Check sheet for the modelled part. Datum: model origin and axes. Units: mm. A direction names the side the tool comes from. Give positions to 0.01 mm unless a question says otherwise; leave off trailing zeros. Write each loop counter-clockwise with the first axis right and the second up, starting at its lowest first coordinate (ties: lowest second). Pieces come first, ordered by that corner, then holes. Notation, with made-up numbers: (30.5, 75.5) -> (42.5, 75.5) arc R21 ccw to (42.5, 88.5) -> close; hole circle Ø4 at (21, 84.25). An arc over 180 degrees is marked (long way). Use a Markdown table: item, result. Add a question column.
1. Cross-section at A-A (x = 15.24). Enter the section's corners in (y, z) (1 decimal).
2. Release check for a two-part mould opening along Y. For faces 1 (the flat face through (15, -3, -0.159)), 2 (the cylindrical face through (0.267, 4.845, 1.526)), 3 (the flat face through (-10.16, 0, 0)) record: released by +Y, released by -Y, zero draft, split by the parting line, or undercut.
3. Scan lines: probe 1 along X at (y, z) = (0, 3.95); probe 2 along X at (y, z) = (-1.9, 0); probe 3 along Z at (x, y) = (17.5, 2.25). Record each from-to range of solid material in increasing order. Write a range as [from, to].
4. Gauge pin test, flat ends, axial feed: P1, Ø4, axis at x = 16.5, y = -3.5, coming from the +Z side; P2, Ø0.6, axis at x = -16.5, y = 0.5, coming from the -Z side; P3, Ø2, axis at x = 10.5, y = -2.5, coming from the -Z side. Record the tip position at first contact, or that the pin passes through.
5. Cross-section at C-C (z = 2.5). Enter the section's corners in (x, y).
6. Set-up check for faces 4 (the flat face through (15, 3, 0.159)), 5 (the flat face through (-14.67, 0.01, -0.891)), 6 (the flat face through (19.05, 0, -3)), 7 (the cylindrical face through (15.187, 0.54, -1.493)): record each of +Z, -Z, +X, -X, +Y, -Y from which the full face is reachable in a straight line by a thin tool's end or side.
7. Cross-section at B-B (y = 2.5). Enter the section's corners in (x, z).
8. Cross-section at D-D (x = 3). Enter the section's corners in (y, z), then the cut area to 3 significant figures.
from build123d import *

# Parameters (mm, degrees)
F0_R      = 5.08
F1_DEPTH  = 19.05
F3_D      = 3.175
F3_DEPTH  = 7.62
F3_TIP    = 0.9538662327
F4_W      = 2.1017943509
F4_H      = 1.7811305588
F5_DEPTH  = 8.89
F7_DEPTH  = 7.62
F9_R      = 0.396875
F10_DEPTH = 17.781
F12_R     = 0.396875
F13_DEPTH = 25.4


with BuildPart() as f1:
    # F0 (on Right) → F1 (new body, symmetric)
    with BuildSketch(Plane.YZ):
        Circle(F0_R)
    extrude(amount=F1_DEPTH, both=True)

    # F3
    with Locations(Plane.YZ.offset(19.05)):
        with Locations((0, 0)):
            Hole(F3_D / 2, depth=F3_DEPTH)
            with Locations((0, 0, -(F3_DEPTH + F3_TIP / 2))):  # 118° drill point
                Cone(0, F3_D / 2, F3_TIP, mode=Mode.SUBTRACT)

    # F4 (on face) → F5 (cut)
    with BuildSketch(Plane(origin=(-19.05, 0, 0), x_dir=(0, -1, 0), z_dir=(-1, 0, 0))):
        Rectangle(F4_W, F4_H)
    extrude(amount=-F5_DEPTH, mode=Mode.SUBTRACT)

    # F6 (on face) → F7 (cut)
    with BuildSketch(Plane.YZ.offset(19.05)):
        with BuildLine():
            ThreePointArc((5.08, 0), (5.0793796935, 0.0793846935), (5.0775189254, 0.15875))
            Line((5.0775189254, 0.15875), (1.5795425564, 0.15875))
            ThreePointArc((1.5795425564, 0.15875), (1.5855093911, 0.0794746554), (1.5875, 0))
            ThreePointArc((1.5875, 0), (1.5855093911, -0.0794746554), (1.5795425564, -0.15875))
            Line((1.5795425564, -0.15875), (5.0775189254, -0.15875))
            ThreePointArc((5.0775189254, -0.15875), (5.0793796935, -0.0793846935), (5.08, 0))
        make_face()
        with BuildLine():
            Line((-1.5795425564, 0.15875), (-5.0775189254, 0.15875))
            ThreePointArc((-5.0775189254, 0.15875), (-5.08, 0), (-5.0775189254, -0.15875))
            Line((-5.0775189254, -0.15875), (-1.5795425564, -0.15875))
            ThreePointArc((-1.5795425564, -0.15875), (-1.5875, 0), (-1.5795425564, 0.15875))
        make_face()
    extrude(amount=-F7_DEPTH, mode=Mode.SUBTRACT)

    # F9 (on offset) → F10 (cut, through all)
    with BuildSketch(Plane.XY.offset(12.7)):
        with Locations((-15.24, 0)):
            Circle(F9_R)
        with Locations((15.24, 0)):
            Circle(F9_R)
    extrude(amount=-F10_DEPTH, mode=Mode.SUBTRACT)

    # F12 (on offset) → F13 (cut)
    with BuildSketch(Plane.XZ.offset(12.7)):
        with Locations((-15.24, 0)):
            Circle(F12_R)
    extrude(amount=-F13_DEPTH, mode=Mode.SUBTRACT)


solid = f1.part
Worked answers:
| question | item | result |
|---|---|---|
| 1 | outline | (-5.1, -0.2) arc R5.1 ccw to (-0.4, -5.1) -> (-0.4, -1.5) arc R1.6 cw to (-1.6, -0.2) -> close; (-5.1, 0.2) -> (-1.6, 0.2) arc R1.6 cw to (-0.4, 1.5) -> (-0.4, 5.1) arc R5.1 ccw to start; (0.4, -5.1) arc R5.1 ccw to (5.1, -0.2) -> (1.6, -0.2) arc R1.6 cw to (0.4, -1.5) -> close; (0.4, 1.5) arc R1.6 cw to (1.6, 0.2) -> (5.1, 0.2) arc R5.1 ccw to (0.4, 5.1) -> close |
| 2 | face 1 | zero draft |
| 2 | face 2 | split by the parting line |
| 2 | face 3 | undercut |
| 3 | probe 1 | x = [-19.05, -15.64], [-14.84, 14.84], [15.64, 19.05] |
| 3 | probe 2 | x = [-19.05, -15.64], [-14.84, 11.43] |
| 3 | probe 3 | z = [-4.55, -0.16], [0.16, 4.55] |
| 4 | P1 | stops at z = 4.85 |
| 4 | P2 | stops at z = -5.08 |
| 4 | P3 | stops at z = -4.85 |
| 5 | outline | (-19.05, -4.42) -> (19.05, -4.42) -> (19.05, 4.42) -> (-19.05, 4.42) -> close; hole circle Ø0.79 at (-15.24, 0); hole circle Ø0.79 at (15.24, 0) |
| 6 | face 4 | +X, +Y, -Y |
| 6 | face 5 | -X |
| 6 | face 6 | +Z, -Z, +X, +Y, -Y |
| 6 | face 7 | +X |
| 7 | outline | (-19.05, -4.42) -> (19.05, -4.42) -> (19.05, -0.16) -> (11.43, -0.16) -> (11.43, 0.16) -> (19.05, 0.16) -> (19.05, 4.42) -> (-19.05, 4.42) -> close; hole circle Ø0.79 at (-15.24, 0) |
| 8 | outline | circle Ø10.16 at (0, 0) |
| 8 | area | 81.1 mm² |
